Part model, mm, in its own coordinate system. A direction names the side the tool comes from. Round coordinates to 2 decimals unless told otherwise and drop trailing zeros. Loops run counter-clockwise (first coordinate to the right, second up) from the corner with the lowest first, then second, coordinate; pieces in that order, holes last.
(1) Probe probe 1 along X at (y, z) = (16, -0.5); probe 2 along X at (y, z) = (17.65, -10); probe 3 along Z at (x, y) = (23, 17.8). List the from-to ranges inside material, lowest first.
(2) Cut at C-C on x = 0. List the corners of the cut face in (y, z).
(3) Flat gauge pins, fed straight in: pin 1 (3 mm diameter, centred on x = 5, z = 12, fed in from +Y); pin 2 (5.5 mm diameter, centred on y = 2.5, z = 2.5, fed in from +X); pin 3 (5 mm diameter, centred on x = 23, z = 10, fed in from -Y). Where does each tip first touch, or does it go through?
(4) Cut at D-D on z = -14.5. List the corners of the cut face in (x, y) (3 decimals), then the cut area to 3 significant figures.
(5) Mould opens along X. For faces 1 (the face through (-22.914, 17.858, -21.934)), 2 (the face through (23, 16.75, -5)), 3 (the face through (18.07, 18.15, -4.75)), 4 (the face through (26, 18, 11)) say: +X half, -X half, draft (parallel to the pull), parting line (faces both ways), or undercut.
(6) Cut at A-A on z = 0. Count the separate pieces of the cut face and the enclosed holes in it, then the cut area to 3 significant figures.
(7) Tool access for faces 5 (the face through (0.22, 4.4, -24.43)), 6 (the face through (-23, 18.75, -5)), 7 (the face through (-18.07, 18.15, -4.75)), 8 (the face through (-2.9, 3, 1)): list every direction of +Z, -Z, +X, -X, +Y, -Y with a clear straight run to the whole face (end or side of a thin tool).
from build123d import *

# Parameters (mm, degrees)
SKETCH2_W           = 35
SKETCH2_H           = 50
BOSS_EXTRUDE1_DEPTH = 5
BOSS_EXTRUDE2_DEPTH = 2
SKETCH4_R           = 1.55
BOSS_EXTRUDE3_DEPTH = 2
FILLET1_R           = 2
FILLET2_R           = 10
CUT_EXTRUDE1_DEPTH  = 40.91088123
CUT_EXTRUDE2_DEPTH  = 56.121529602


# Some blends are built 0.0001 mm under size
with BuildPart() as part:
    # Sketch2 → Boss-Extrude1 (new body)
    with BuildSketch(Plane(origin=(0, 0, 0), x_dir=(1, 0, 0), z_dir=(0, 1, 0))):
        Rectangle(SKETCH2_W, SKETCH2_H)
    extrude(amount=BOSS_EXTRUDE1_DEPTH)

    # Sketch3 → Boss-Extrude2 (add)
    with BuildSketch(Plane(origin=(17.5, 0, 0), x_dir=(0, 0, -1), z_dir=(1, 0, 0))):
        Polygon((-25, 0), (-15, 18.75), (25, 18.75), (25, 0), align=None)
    boss_extrude2 = extrude(amount=BOSS_EXTRUDE2_DEPTH)

    # Mirror1: Boss-Extrude2 across plane
    add(boss_extrude2.mirror(Plane(origin=(0, 0, 0), x_dir=(0, 0, 1), z_dir=(1, 0, 0))))

    # Sketch4 → Boss-Extrude3 (add)
    with BuildSketch(Plane(origin=(0, 18.75, 0), x_dir=(1, 0, 0), z_dir=(0, 1, 0))):
        Polygon((-19.5, -15), (-29.5, -15), (-23.5, 25), (-19.5, 25), align=None)
        with Locations(Location((-23, -10, 0), (0, 0, 270))):
            Circle(SKETCH4_R, mode=Mode.SUBTRACT)
        with Locations(Location((-23, 0, 0), (0, 0, 270))):
            Circle(SKETCH4_R, mode=Mode.SUBTRACT)
        with Locations(Location((-23, 10, 0), (0, 0, 270))):
            Circle(SKETCH4_R, mode=Mode.SUBTRACT)
    boss_extrude3 = extrude(amount=-BOSS_EXTRUDE3_DEPTH)

    # Fillet1
    fillet1_edges = [part.edges().sort_by_distance(p)[0] for p in [
        (-17.5, 5, -1.333333333),
        (17.5, 5, -1.333333333),
        (17.5, 18.75, -5),
        (19.5, 0, 0),
        (-17.5, 11.875, -25),
        (-17.5, 18.75, -5),
        (-19.5, 0, 0),
        (17.5, 11.875, -25),
        (0, 0, -25),
        (0, 5, -25),
    ]]
    fillet(fillet1_edges, radius=FILLET1_R - 0.0001)  # a hair under: the kernel refuses the full size

    # Mirror2: Boss-Extrude3 across plane
    add(boss_extrude3.mirror(Plane(origin=(0, 0, 0), x_dir=(0, 0, 1), z_dir=(1, 0, 0))))

    # Fillet2
    # the kernel refuses this fillet: 10 mm, written as the material it takes off along each edge
    with BuildSketch(Plane(origin=(-29.5, 47.456981223, 15), x_dir=(1, 0, 0), z_dir=(0, -1, 0))) as fillet2_piece_1:
        with BuildLine():
            CenterArc((11.592726167, -9.872346396), FILLET2_R, 99.164678829, 89.366086781)
            Line((1.703362639, -11.355750925), (0, 0))
            Line((0, 0), (10, 0))
        make_face()
    extrude(amount=59.413962446, mode=Mode.SUBTRACT)
    with BuildSketch(Plane(origin=(29.5, 47.456981223, 15), x_dir=(-0.1483404529302447, 0, -0.9889363528682975), z_dir=(0, -1, 0))) as fillet2_piece_2:
        with BuildLine():
            CenterArc((11.482792489, -10), FILLET2_R, 90, 89.366086781)
            Line((1.483404529, -9.889363529), (0, 0))
            Line((0, 0), (11.482792489, 0))
        make_face()
    extrude(amount=59.413962446, mode=Mode.SUBTRACT)
    with BuildSketch(Plane(origin=(-23.5, 37.183288466, -25), x_dir=(1.0, 0, 1.2229911091485247e-12), z_dir=(0, -1, 0))) as fillet2_piece_3:
        with BuildLine():
            CenterArc((8.795602585, 8.775144156), FILLET2_R, 188.53076561, 52.813201583)
            Line((-1.093760944, 7.291739627), (0, 0))
            Line((0, 0), (4.0001, 0))
        make_face()
    extrude(amount=38.866576932, mode=Mode.SUBTRACT)
    with BuildSketch(Plane(origin=(23.5, 37.183288466, -25), x_dir=(-1.0, 0, 1.2229911091485247e-12), z_dir=(0, -1, 0))) as fillet2_piece_4:
        with BuildLine():
            CenterArc((8.795602585, -8.775144156), FILLET2_R, 118.656032807, 52.813201583)
            Line((-1.093760944, -7.291739627), (0, 0))
            Line((0, 0), (4.0001, 0))
        make_face()
    extrude(amount=38.866576932, mode=Mode.SUBTRACT)

    # Sketch5 → Cut-Extrude1 (cut, through all)
    with BuildSketch(Plane(origin=(0, 5, 0), x_dir=(1, 0, 0), z_dir=(0, 1, 0))):
        with BuildLine():
            Line((2.9, 18), (2.9, -20))
            ThreePointArc((2.9, -20), (0, -22.9), (-2.9, -20))
            Line((-2.9, -20), (-2.9, 18))
            ThreePointArc((-2.9, 18), (0, 20.9), (2.9, 18))
        make_face()
    extrude(amount=-CUT_EXTRUDE1_DEPTH, mode=Mode.SUBTRACT)

    # Sketch6 → Cut-Extrude2 (cut, through all)
    with BuildSketch(Plane.ZY.offset(17.5)):
        Polygon((25, 5), (22.333333333, 5), (25, 0), align=None)
    extrude(amount=-CUT_EXTRUDE2_DEPTH, mode=Mode.SUBTRACT)


solid = part.part
Final values:
1. probe 1: x = -19.5 to -17.5, 17.5 to 19.5
1. probe 2: x = -25.75 to -24.55, -21.45 to -17.71, 17.71 to 21.45, 24.55 to 25.75
1. probe 3: z = -21.81 to -11.55, -8.45 to -1.55, 1.55 to 8.45, 11.55 to 13.73
2. outline: (0, -23) arc R2 ccw to (2, -25) - (3, -25) arc R2 ccw to (5, -23) - (5, -20.9) - (0, -20.9) - close; (0, 22.9) - (3.94, 22.9) - (0, 25) - close
3. pin 1: stops at y = 5
3. pin 2: stops at x = 19.5
3. pin 3: stops at y = 16.75
4. outline: (-25.075, 16.75) - (-19.5, 16.75) - (-19.5, 2) arc R2 ccw to (-17.5, 0) - (-2.9, 0) - (-2.9, 5) - (-15.5, 5) arc R2 cw to (-17.5, 7) - (-17.5, 16.75) arc R2 ccw to (-19.5, 18.75) - (-25.075, 18.75) - close; (2.9, 0) - (17.5, 0) arc R2 ccw to (19.5, 2) - (19.5, 16.75) - (25.075, 16.75) - (25.075, 18.75) - (19.5, 18.75) arc R2 ccw to (17.5, 16.75) - (17.5, 7) arc R2 cw to (15.5, 5) - (2.9, 5) - close
4. area: 242 mm2
5. face 1: -X half
5. face 2: draft
5. face 3: undercut
5. face 4: +X half
6. separate pieces: 4
6. enclosed holes: 0
6. area: 238 mm2
7. face 5: -Z, +Y
7. face 6: +Z, -Z, +X, -X, +Y
7. face 7: +Z, -Z, +Y
7. face 8: +Y, -Y
